For this review, use the dimensioned drawing (mm, ordinates from the lowest corner) and the shaded views. Give positions to 0.01 mm unless a question says otherwise; leave off trailing zeros. Loops run counter-clockwise (first coordinate to the right, second up) from the corner with the lowest first, then second, coordinate; pieces in that order, holes last. Notation, with made-up numbers: M -5,-6.5 L 41,-6.5 A16 cw 41,8.5 Z; hole C 34,1.5 d4. An arc over 180 degrees is marked long. Use a Markdown table: item, result. Add a question column.
(1) Add section B-B, the plane y = 27. Give the boundary of the cut face in (x, z).
(2) For probe 1 along X at (y, z) = (34, 22.5); probe 2 along Z at (x, y) = (96, 36.5), list the stretches that pass through material, from the lowest coordinate up.
(3) Draft analysis for pull direction X (two halves, no side actions). For the marked faces 1, 2, 3 and 4, state which applies: pulls with the +X half, pulls with the -X half, needs draft (parallel to the pull), parting line crosses it, or undercut.
(4) Add section C-C, the plane x = 29. Give the boundary of the cut face in (y, z) (3 decimals), then the cut area to 3 significant figures.
(5) Add section A-A, the plane z = 22.5. Give the boundary of the cut face in (x, y).
(6) Insertion check: pin 1 Ø12 at (x, y) = (68.5, 28.5) entering from -Z; pin 2 Ø2 at (y, z) = (56.5, 21) entering from -X; pin 3 Ø6 at (x, y) = (85.5, 31.5) entering from +Z; pin 4 Ø6 at (x, z) = (123, 29.5) entering from -Y. Each pin has a flat end and moves straight along its axis. Give the tip position at first contact, or say it passes through.
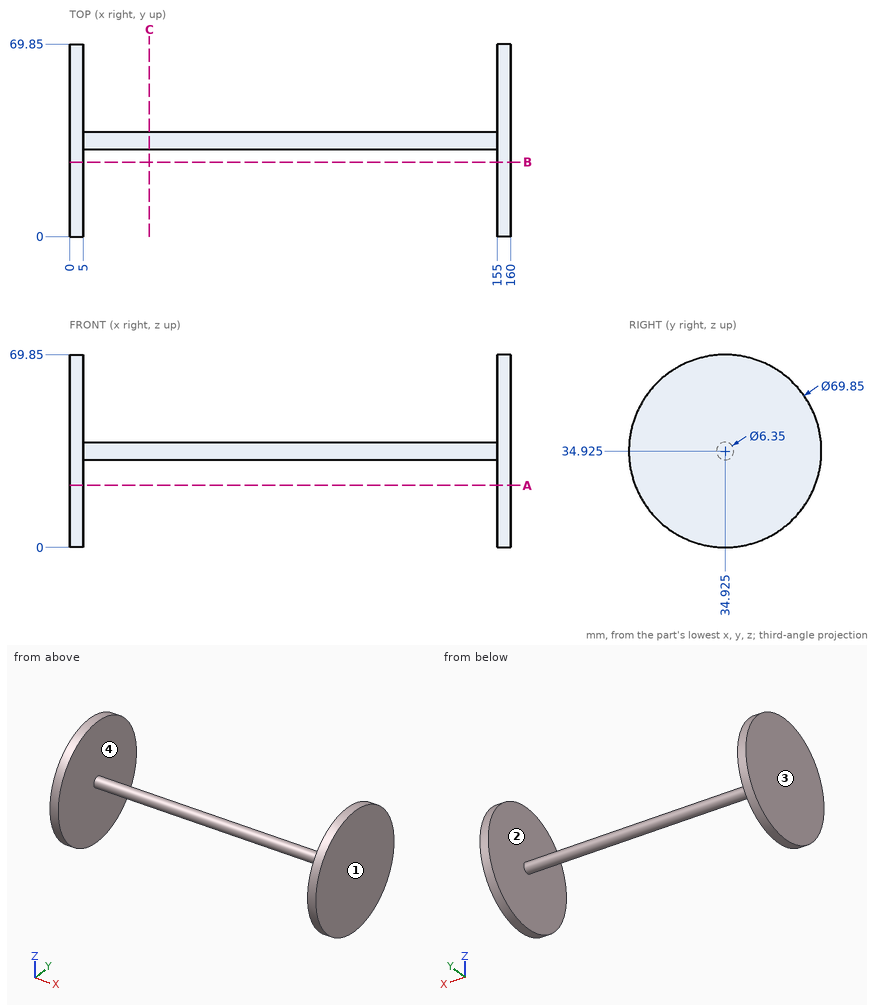
Established:
| question | item | result |
|---|---|---|
| 1 | outline | M 0,0.91 L 5,0.91 L 5,68.94 L 0,68.94 Z; M 155,0.91 L 160,0.91 L 160,68.94 L 155,68.94 Z |
| 2 | probe 1 | 0 to 5, 155 to 160 |
| 2 | probe 2 | 32.17 to 37.68 |
| 3 | face 1 | pulls with the +X half |
| 3 | face 2 | undercut |
| 3 | face 3 | pulls with the -X half |
| 3 | face 4 | undercut |
| 4 | outline | C 34.925,34.925 d6.35 |
| 4 | area | 31.7 mm^2 |
| 5 | outline | M 0,2.28 L 5,2.28 L 5,67.57 L 0,67.57 Z; M 155,2.28 L 160,2.28 L 160,67.57 L 155,67.57 Z |
| 6 | pin 1 | z = 31.78 |
| 6 | pin 2 | x = 0 |
| 6 | pin 3 | z = 38.07 |
| 6 | pin 4 | y = 32.88 |
